Model file for the job. Use its own axes, mm. Face numbers are marked on the shaded views. A direction names the side the tool comes from. Round coordinates to 2 decimals unless told otherwise and drop trailing zeros. Order: outer loops, then holes, each group sorted by start corner. A loop starts at its lowest first (then second) coordinate and runs counter-clockwise, first axis right, second up. Notation, with made-up numbers: (56.5, 64) - (67.5, 64) arc R27 ccw to (67.5, 91) - close; hole circle Ø7 at (-24, -39.75). An arc over 180 degrees is marked (long way). Write item = value, one per line.
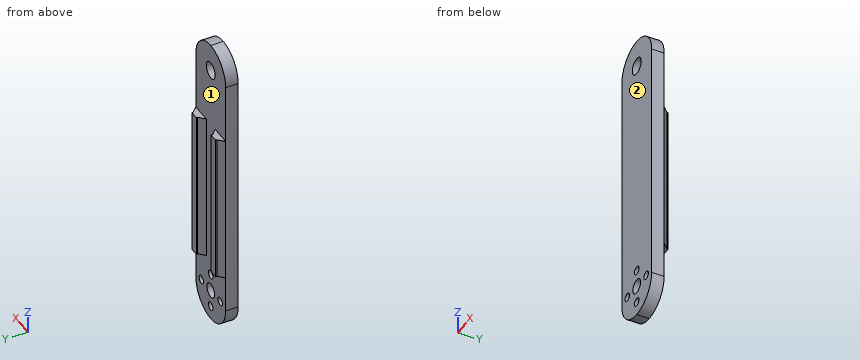
Autodesk Inventor part; units mm, degrees
ref_plane "YZ Plane" through (0, 0, 0) normal (1, 0, 0) x (0, 1, 0)
ref_plane "XZ Plane" through (0, 0, 0) normal (0, 1, 0) x (-1, 0, 0)
ref_plane "XY Plane" through (0, 0, 0) normal (0, 0, 1) x (1, 0, 0)
sketch "Szkic1" plane through (0, 0, 0) normal (0, 1, 0) x (-1, 0, 0)
  line L0 (10, 55) -> (-10, 55)
  line L1 (-10, 55) -> (-10, -55)
  line L2 (-10, -55) -> (10, -55)
  line L3 (10, -55) -> (10, 55)
  line L4 (10, 55) -> (-10, -55) construction
  line L5 (-10, 55) -> (10, -55) construction
  circle A0 centre (0, -43.65) radius 2.6
  circle A1 centre (0, -37.3) radius 1.5
  circle A2 centre (0, -50) radius 1.5
  circle A3 centre (-6.35, -43.65) radius 1.5
  circle A4 centre (6.35, -43.65) radius 1.5
  line L6 (6.35, -43.65) -> (-6.35, -43.65)
  line L7 (0, -37.3) -> (0, -50)
  point P0 (0, 0)
  dimension "d0" = 20
  dimension "d1" = 110
  dimension "d2" = 5.2
  dimension "d3" = 3
  dimension "d4" = 3
  dimension "d5" = 6.35
  dimension "d6" = 6.35
  dimension "d7" = 5
  dimension "d22" = 3
  dimension "d23" = 3
  dimension "d24" = 6.35
  dimension "d25" = 6.35
  dimension "d26" = 8.9803
  dimension "d27" = 8.9803
  dimension "d28" = 3.65
extrude "Wyciągnięcie proste1" add sketch "Szkic1" along normal blind 4.5 contours L3 L2 L1 L0 | A3 | A4
sketch "Szkic3" plane through (0, 4.5, 0) normal (0, 1, 0) x (1, 0, 0)
  circle A0 centre (0, -45) radius 2.5
  circle A1 centre (0, -45) radius 2.5
  point P0 (0, 0)
fillet "Zaokrąglenie1" radius 10 4 edges at (10, 2.25, -55) (-10, 2.25, -55) (10, 2.25, 55) (-10, 2.25, 55)
extrude "Wyciągnięcie proste4" cut sketch "Szkic3" against normal blind 10
sketch "Szkic4" plane through (0, 4.5, 0) normal (0, 1, 0) x (1, 0, 0)
  circle A0 centre (0, -45) radius 2.5
  circle A1 centre (0, -45) radius 3
  point P0 (0, 0)
  dimension "d19" = 6
extrude "Wyciągnięcie proste5" cut sketch "Szkic4" against normal blind 10
extrude "Wyciągnięcie proste6" cut sketch "Szkic1" along normal blind 7 contours A3 | A4
sketch "Szkic5" plane through (0, 4.5, 0) normal (0, 1, 0) x (1, 0, 0)
  line L0 (-8, -23.35) -> (-5, -23.35)
  line L1 (-5, -23.35) -> (-5, 31.65)
  line L2 (-5, 31.65) -> (-8, 31.65)
  line L3 (-8, 31.65) -> (-8, -23.35)
  line L4 (5, -23.35) -> (8, -23.35)
  line L5 (8, -23.35) -> (8, 31.65)
  line L6 (8, 31.65) -> (5, 31.65)
  line L7 (5, 31.65) -> (5, -23.35)
  circle A0 centre (0, 43.65) radius 2.6
  line L8 (10, -45) -> (10, 45)
  line L9 (-10, 45) -> (-10, -45)
  point P0 (0, 0)
  point P1 (6.5, 31.65)
  point P2 (6.5, -23.35)
  point P3 (-6.5, 31.65)
  point P4 (-6.5, -23.35)
  dimension "d31" = 55
  dimension "d32" = 55
  dimension "d33" = 67
  dimension "d34" = 3
  dimension "d35" = 3
  dimension "d36" = 2
  dimension "d37" = 2
extrude "Wyciągnięcie proste7" add sketch "Szkic5" along normal blind 2.5 contours L3 L2 L1 L0 | L7 L6 L5 L4
chamfer "Faza1" distance 2 angle 45 4 edges at (8, 4.5, -4.15) (-5, 4.5, -4.15) (-8, 4.5, -4.15) (5, 4.5, -4.15)
properties part number "link1_print_Drukowanie 3D"
1) Cut at A-A (z = -37.3). Write the cut outline in (x, y).
Conclusion:
outline = (-10, 0) - (-1.5, 0) - (-1.5, 4.5) - (-10, 4.5) - close; (1.5, 0) - (10, 0) - (10, 4.5) - (1.5, 4.5) - close
2) Wall check: line 1 along Z through (x, y) = (0, 2.1); line 2 along X through (y, z) = (1.85, -43.65); line 3 along Z through (x, y) = (1.25, 3). Give the ranges that are in metal, low to high.
Conclusion:
line_1 = -55 to -51.5, -48.5 to -46.25, -41.05 to -38.8, -35.8 to 42, 48 to 55
line_2 = -10 to -7.85, -4.85 to -2.6, 2.6 to 4.85, 7.85 to 10
line_3 = -54.92 to -50.83, -49.17 to -45.93, -41.37 to -38.13, -36.47 to 42.27, 47.73 to 54.92
3) Cut at C-C (x = 6). Write the cut outline in (y, z).
Conclusion:
outline = (0, -53) - (4.5, -53) - (4.5, -45.11) - (0, -45.11) - close; (0, -42.19) - (4.5, -42.19) - (4.5, -31.65) - (7, -31.65) - (7, 23.35) - (4.5, 23.35) - (4.5, 53) - (0, 53) - close
4) 3-axis set-ups, long thin cutter, end or side, ignore diameter. For the marked faces 1 and 2: which of +Z, -Z, +X, -X, +Y, -Y reach the whole face in a straight line?
Conclusion:
face_1 = +Y
face_2 = +Z, -Z, +X, -X, -Y
5) Cut at B-B (y = 3). Give the number of separate pieces and of enclosed holes in the cut face, and give its area (3 significant figures).
Conclusion:
separate_pieces = 1
enclosed_holes = 6
area = 2,040 mm^2
6) Flat gauge pins, fed straight in: pin 1 Ø1.2 at (x, y) = (-6.5, 6) entering from -Z; pin 2 Ø4 at (x, z) = (6.35, -43.65) entering from +Y; pin 3 Ø1.8 at (x, z) = (-6.35, -43.65) entering from +Y; pin 4 Ø4 at (x, y) = (-6, 3) entering from +Z. Where does each tip first touch, or does it go through?
Conclusion:
pin_1 = -31.65
pin_2 = 4.5
pin_3 = through
pin_4 = 54.17
